The figure shows three views and two pictorial views of one solid part (mm, origin at its lowest corner). Answer the questions. A direction names the side the tool comes from. Give positions to 0.01 mm unless a question says otherwise; leave off trailing zeros. Write each loop counter-clockwise with the first axis right and the second up, starting at its lowest first coordinate (ties: lowest second). Pieces come first, ordered by that corner, then holes. Notation, with made-up numbers: M -37,57.5 L 11,57.5 A25 cw 11,91.5 Z; hole C -32,-24.5 d8. An arc over 180 degrees is marked long. Return JSON: item names as keys, results as strings.
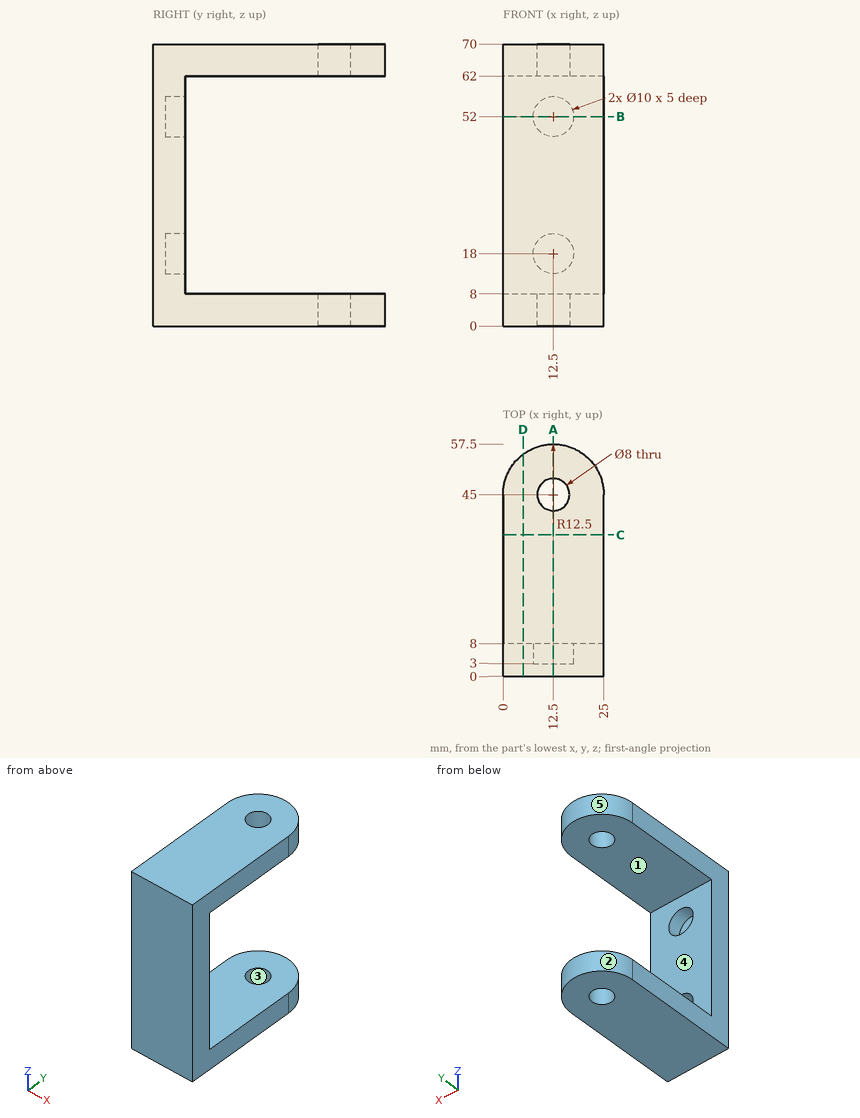
Item 1: Given pin 1 Ø8 at (x, y) = (4, 28.5) entering from -Z; pin 2 Ø12 at (x, z) = (12.5, 28) entering from +Y; pin 3 Ø10 at (y, z) = (20, 16.5) entering from -X; pin 4 Ø9 at (x, z) = (12.5, 52) entering from +Y, each flat-ended and moving along its own axis, determine where each tip first touches the part or whether it passes through.
Geometry results:
{"pin 1": "stops at z = 0", "pin 2": "stops at y = 8", "pin 3": "passes through", "pin 4": "stops at y = 3"}
Item 2: A cutting plane is placed at C-C, the plane y = 35. Write down the section's boundary in (x, z).
Geometry results:
{"outline": "M 0,0 L 25,0 L 25,8 L 0,8 Z; M 0,62 L 25,62 L 25,70 L 0,70 Z"}
Item 3: Find the intervals of material crossed by line 1 (Z direction, x = 12.5, y = 6.35); line 2 (Z direction, x = 3.5, y = 16); line 3 (Y direction, x = 14.75, z = 55), in increasing order.
Geometry results:
{"line 1": "z = 0 to 13, 23 to 47, 57 to 70", "line 2": "z = 0 to 8, 62 to 70", "line 3": "y = 0 to 3"}
Item 4: Determine the mould class of the marked faces 1, 2 and 3 for opening direction Y: +Y half, -Y half, draft (parallel to the pull), parting line (faces both ways), or undercut.
Geometry results:
{"face 1": "draft", "face 2": "+Y half", "face 3": "undercut"}
Item 5: A cutting plane is placed at D-D, the plane x = 5. Write down the section's boundary in (y, z), plus the area to 3 significant figures.
Geometry results:
{"outline": "M 0,0 L 55,0 L 55,8 L 8,8 L 8,62 L 55,62 L 55,70 L 0,70 Z", "area": "1,310 mm2"}
Item 6: A cutting plane is placed at A-A, the plane x = 12.5. Write down the section's boundary in (y, z), plus the area to 3 significant figures.
Geometry results:
{"outline": "M 0,0 L 41,0 L 41,8 L 8,8 L 8,13 L 3,13 L 3,23 L 8,23 L 8,47 L 3,47 L 3,57 L 8,57 L 8,62 L 41,62 L 41,70 L 0,70 Z; M 49,0 L 57.5,0 L 57.5,8 L 49,8 Z; M 49,62 L 57.5,62 L 57.5,70 L 49,70 Z", "area": "1,120 mm2"}
Item 7: A cutting plane is placed at B-B, the plane z = 52. Write down the section's boundary in (x, y).
Geometry results:
{"outline": "M 0,0 L 25,0 L 25,8 L 17.5,8 L 17.5,3 L 7.5,3 L 7.5,8 L 0,8 Z"}
Item 8: Which of the six approach directions +Z, -Z, +X, -X, +Y, -Y give full straight-line access (tool end or side, diameter ignored) to the marked faces 4 and 5?
Geometry results:
{"face 4": "+X, -X, +Y", "face 5": "+Z, -Z, +Y"}
